```python
from build123d import *

# Parameters (mm, degrees)
SKETCH_1_R          = 4.5
EXTRUDE_1_DEPTH     = 55
EXTRUDE_2_DEPTH     = 15
SKETCH_4_R          = 2
CUT_EXTRUDE_1_DEPTH = 71.544312315
CUT_EXTRUDE_3_DEPTH = 71.544312315
FILLET_1_R          = 0.5
SKETCH1_R           = 4.5
CUT_EXTRUDE1_DEPTH  = 20


with BuildPart() as part:
    # 草图1 → 凸台-拉伸1 (new body)
    with BuildSketch(Plane(origin=(0, 0, 0), x_dir=(1, 0, 0), z_dir=(0, 1, 0))):
        with Locations(Location((0, 0, 0), (0, 0, 270))):
            Circle(SKETCH_1_R)
    extrude(amount=EXTRUDE_1_DEPTH)

    # 草图2 → 凸台-拉伸2 (add)
    with BuildSketch(Plane(origin=(0, 55, 0), x_dir=(1, 0, 0), z_dir=(0, 1, 0))):
        with BuildLine():
            Line((-3, 3.010398645), (-3, -3.010398645))
            ThreePointArc((-3, -3.010398645), (0, -4.25), (3, -3.010398645))
            Line((3, -3.010398645), (3, 3.010398645))
            ThreePointArc((3, 3.010398645), (0, 4.25), (-3, 3.010398645))
        make_face()
    extrude(amount=EXTRUDE_2_DEPTH)

    # 草图4 → 切除-拉伸1 (cut, through all)
    with BuildSketch(Plane.ZY.offset(3)):
        with Locations((0, 61.5)):
            Circle(SKETCH_4_R)
    extrude(amount=-CUT_EXTRUDE_1_DEPTH, mode=Mode.SUBTRACT)

    # 草图5 → 切除-拉伸3 (cut, through all)
    with BuildSketch(Plane.ZY.offset(3)):
        with BuildLine():
            Line((-4.813255022, 64.251745482), (-4.813255022, 72.406434262))
            Line((-4.813255022, 72.406434262), (5.466876832, 72.406434262))
            Line((5.466876832, 72.406434262), (5.466876832, 63.634516306))
            ThreePointArc((5.466876832, 63.634516306), (0.449497866, 65.986517994), (-4.813255022, 64.251745482))
        make_face()
    extrude(amount=-CUT_EXTRUDE_3_DEPTH, mode=Mode.SUBTRACT)

    # 圆角1
    fillet_1_edges = [part.edges().sort_by_distance(p)[0] for p in [
        (0, 64.679603547, -4.25),
        (0, 64.679603547, 4.25),
    ]]
    fillet(fillet_1_edges, radius=FILLET_1_R)

    # Sketch1 → Cut-Extrude1 (cut)
    with BuildSketch(Plane.XZ):
        with Locations(Location((0, 0, 0), (0, 0, 270))):
            Circle(SKETCH1_R)
    extrude(amount=-CUT_EXTRUDE1_DEPTH, mode=Mode.SUBTRACT)


solid = part.part
```
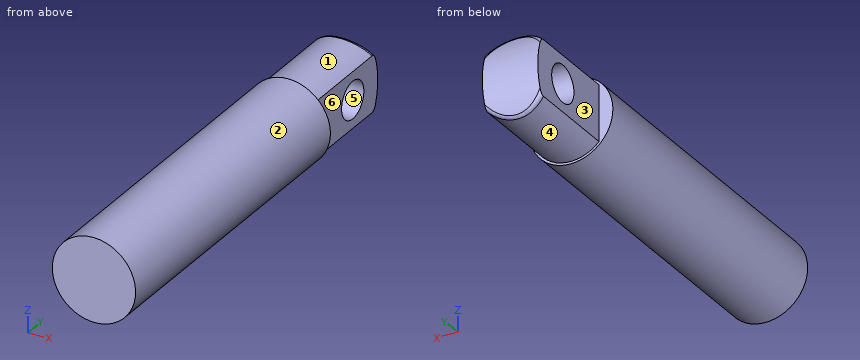
Verification items for the finished model (mm, model axes). Face numbers are marked on the shaded views. A direction names the side the tool comes from. Coordinates: 2 decimals unless noted, no trailing zeros. Order: outer loops, then holes, each group sorted by start corner. A loop starts at its lowest first (then second) coordinate and runs counter-clockwise, first axis right, second up. Notation, with made-up numbers: (59.5, 86.25) -> (118.5, 86.25) arc R9 ccw to (118.5, 94.25) -> close; hole circle Ø10 at (-40, 81). An arc over 180 degrees is marked (long way). Answer as CSV lines item,"result". Start each with the question number.
1) Cross-section at B-B, the plane z = 0. Record the boundary of the cut face in (x, y), then the cut area to 3 significant figures.
2) Cross-section at A-A, the plane y = 61.5. Record the boundary of the cut face in (x, z), then the cut area to 3 significant figures.
3) Set-up check for the marked faces 1, 2 and 3: record each of +Z, -Z, +X, -X, +Y, -Y from which the full face is reachable in a straight line by a thin tool's end or side.
4) Cross-section at C-C, the plane y = 24. Record the boundary of the cut face in (x, z), then the cut area to 3 significant figures.
5) Cross-section at D-D, the plane x = 3.5. Record the boundary of the cut face in (y, z).
6) Material ranges on L1, parallel to Y at x = 1.85, z = 0; L2, parallel to X at y = 58.5, z = -2.25; L3, parallel to X at y = 52, z = 0.25, recorded low to high. Write a range as [from, to].
7) Release check for a two-part mould opening along Z. For the marked faces 4, 5 and 6 record: released by +Z, released by -Z, zero draft, split by the parting line, or undercut.
8) Gauge pin test, flat ends, axial feed: pin 1 Ø3 at (y, z) = (55, -2.5) entering from +X; pin 2 Ø3 at (y, z) = (61.5, 0) entering from -X; pin 3 Ø1.5 at (x, y) = (-3.5, 43) entering from +Z. Record the tip position at first contact, or that the pin passes through.
Conclusion:
1,outline,"(-4.5, 20) -> (4.5, 20) -> (4.5, 55) -> (3, 55) -> (3, 59.5) -> (-3, 59.5) -> (-3, 55) -> (-4.5, 55) -> close; (-3, 63.5) -> (3, 63.5) -> (3, 66) -> (-3, 66) -> close"
1,area,"357 mm²"
2,outline,"(-3, -3.01) arc R4.25 ccw to (3, -3.01) -> (3, -2) -> (-3, -2) -> close; (-3, 2) -> (3, 2) -> (3, 3.01) arc R4.25 ccw to (-3, 3.01) -> close"
2,area,"22.4 mm²"
3,face 1,"+Z, +Y"
3,face 2,"+Y, -Y"
3,face 3,"+Z, -Z, -X, +Y"
4,outline,"circle Ø9 at (0, 0)"
4,area,"63.6 mm²"
5,outline,"(20, -2.83) -> (55, -2.83) -> (55, 2.83) -> (20, 2.83) -> close"
6,L1,"y = [20, 59.5], [63.5, 66]"
6,L2,"x = [-3, 3]"
6,L3,"x = [-4.49, 4.49]"
7,face 4,"released by -Z"
7,face 5,"undercut"
7,face 6,"zero draft"
8,pin 1,"stops at x = 4.39"
8,pin 2,"passes through"
8,pin 3,"stops at z = 3.56"
